from build123d import *


with BuildPart() as part:
    # Esquisse1 → Révolution1 (revolve)
    with BuildSketch(Plane.XY):
        with BuildLine():
            Line((0, 0), (38, 0))
            ThreePointArc((38, 0), (39.414213562, 0.585786438), (40, 2))
            Line((40, 2), (40, 61.343145751))
            ThreePointArc((40, 61.343145751), (39.847759065, 62.108512615), (39.414213562, 62.757359313))
            Line((39.414213562, 62.757359313), (33.585786438, 68.585786438))
            ThreePointArc((33.585786438, 68.585786438), (33.152240935, 69.234633135), (33, 70))
            Line((33, 70), (33, 80))
            Line((33, 80), (30, 80))
            Line((30, 80), (30, 67))
            ThreePointArc((30, 67), (30.152240935, 66.234633135), (30.585786438, 65.585786438))
            Line((30.585786438, 65.585786438), (36.414213562, 59.757359313))
            ThreePointArc((36.414213562, 59.757359313), (36.847759065, 59.108512615), (37, 58.343145751))
            Line((37, 58.343145751), (37, 5))
            ThreePointArc((37, 5), (36.414213562, 3.585786438), (35, 3))
            Line((35, 3), (0, 3))
            Line((0, 3), (0, 0))
        make_face()
    revolve(axis=Axis((0, 0, 0), (0, 1, 0)))


solid = part.part
Verification items for the finished model (mm, model axes). A direction names the side the tool comes from. Coordinates: 2 decimals unless noted, no trailing zeros. Order: outer loops, then holes, each group sorted by start corner. A loop starts at its lowest first (then second) coordinate and runs counter-clockwise, first axis right, second up. Notation, with made-up numbers: M 0,-16 L 40,-16 A27 ccw 40,2 Z; hole C 43.25,26.25 d8. An arc over 180 degrees is marked long. One line per item, written item: value. Start each with the question number.
Item 1: Sectioned sample at A-A on x = 0. Record the cut outline in (y, z).
Item 2: Sectioned sample at B-B on y = 39. Record the cut outline in (x, z), then the cut area to 3 significant figures.
Item 3: Depth check by flat-ended pin: P1, Ø4, axis at y = 22.5, z = 7.5, coming from the -X side; P2, Ø1, axis at x = -2, y = 27.5, coming from the +Z side; P3, Ø4, axis at x = -25, y = 36, coming from the -Z side. Enter the tip coordinate at first touch or a pass-through.
Item 4: Mould release check, pull along X, two halves, no side actions. Record for faces 1 (the conical face through (-26.88, 68.3, 20.61)), 2 (the flat face through (15, 80, 27)), 3 (the conical face through (29.52, 65.22, -9.3)): pulls with the +X half, pulls with the -X half, needs draft (parallel to the pull), parting line crosses it, or undercut.
Item 5: Access from +Z, -Z, +X, -X, +Y, -Y to the whole of each face (thin tool, end or side, straight path). Record for faces 4 (the flat face through (1, 0, -1)), 5 (the flat face through (0, 3, 0)), 6 (the cylindrical face through (-29.97, 73.41, -1.32)).
Item 6: Thickness scan on probe 1 along Z at (x, y) = (0, 73.75); probe 2 along Y at (x, z) = (-0.5, 25). Record the ranges inside material, lowest first.
Calculated:
1. outline: M 0,-38 A2 ccw 2,-40 L 61.34,-40 A2 ccw 62.76,-39.41 L 68.59,-33.59 A2 cw 70,-33 L 80,-33 L 80,-30 L 67,-30 A2 ccw 65.59,-30.59 L 59.76,-36.41 A2 cw 58.34,-37 L 5,-37 A2 cw 3,-35 L 3,35 A2 cw 5,37 L 58.34,37 A2 cw 59.76,36.41 L 65.59,30.59 A2 ccw 67,30 L 80,30 L 80,33 L 70,33 A2 cw 68.59,33.59 L 62.76,39.41 A2 ccw 61.34,40 L 2,40 A2 ccw 0,38 Z
2. outline: C 0,0 d80; hole C 0,0 d74
2. area: 726 mm^2
3. P1: x = -39.62
3. P2: z = 39.97
3. P3: z = -32.73
4. face 1: parting line crosses it
4. face 2: needs draft
4. face 3: undercut
5. face 4: +Z, -Z, +X, -X, -Y
5. face 5: none
5. face 6: +Y
6. probe 1: -33 to -30, 30 to 33
6. probe 2: 0 to 3
